from build123d import *

# Parameters (mm, degrees)
F1_DEPTH = 14.224
F2_DEPTH = 7.874
F3_DEPTH = 12.7


with BuildPart() as f1:
    # F0 (on Front) → F1 (new body, symmetric)
    with BuildSketch(Plane.XZ):
        Polygon((22.958146, 14.2875), (-45.974, 14.2875), (-52.324, 14.2875), (-52.324, -14.2875), (-45.974, -14.2875), (22.958146, -14.2875), align=None)
    extrude(amount=F1_DEPTH, both=True)

    # F0 (on Front) → F2 (join, symmetric)
    with BuildSketch(Plane.XZ):
        Polygon((17.272, 25.2095), (17.272, 42.7355), (-45.974, 42.7355), (-45.974, 14.2875), (22.958146, 14.2875), (32.52297, 14.2875), (40.125151, 25.2095), align=None)
        with BuildLine():
            Line((0, 22.1615), (-21.336, 22.1615))
            ThreePointArc((-21.336, 22.1615), (-27.686, 28.5115), (-21.336, 34.8615))
            Line((-21.336, 34.8615), (0, 34.8615))
            ThreePointArc((0, 34.8615), (6.35, 28.5115), (0, 22.1615))
        make_face(mode=Mode.SUBTRACT)
        Polygon((32.52297, -14.2875), (22.958146, -14.2875), (-45.974, -14.2875), (-45.974, -42.7355), (17.272, -42.7355), (17.272, -25.365404), (40.233667, -25.365404), align=None)
        with BuildLine():
            Line((0, -34.8615), (-21.336, -34.8615))
            ThreePointArc((-21.336, -34.8615), (-27.686, -28.5115), (-21.336, -22.1615))
            Line((-21.336, -22.1615), (0, -22.1615))
            ThreePointArc((0, -22.1615), (6.35, -28.5115), (0, -34.8615))
        make_face(mode=Mode.SUBTRACT)
    extrude(amount=F2_DEPTH, both=True)

    # F0 (on Front) → F3 (join, symmetric)
    with BuildSketch(Plane.XZ):
        Polygon((40.125151, 25.2095), (52.324, 42.7355), (17.272, 42.7355), (17.272, 25.2095), align=None)
        Polygon((52.324, -42.7355), (40.233667, -25.365404), (17.272, -25.365404), (17.272, -42.7355), align=None)
    extrude(amount=F3_DEPTH, both=True)


solid = f1.part
Design review of the part built by this model. Coordinates are the model's own, in mm. A direction names the side the tool comes from. Give positions to 0.01 mm unless a question says otherwise; leave off trailing zeros. Loops run counter-clockwise (first coordinate to the right, second up) from the corner with the lowest first, then second, coordinate; pieces in that order, holes last. Notation, with made-up numbers: M -39,71 L 12,71 A6 cw 12,76 Z; hole C 76,62.25 d10. An arc over 180 degrees is marked long. Write item = value, one per line.
Q1. We need section A-A (x = 30.5). Give the boundary of the cut face in (y, z), plus the area to 3 significant figures.
Output values:
outline = M -12.7,-42.74 L 12.7,-42.74 L 12.7,-25.37 L 7.87,-25.37 L 7.87,-14.29 L -7.87,-14.29 L -7.87,-25.37 L -12.7,-25.37 Z; M -12.7,25.21 L -7.87,25.21 L -7.87,14.29 L 7.87,14.29 L 7.87,25.21 L 12.7,25.21 L 12.7,42.74 L -12.7,42.74 Z
area = 1,230 mm^2
Q2. To check wall thickness, follow line 1 (Z direction, x = -20, y = 5.5); line 2 (Z direction, x = 35, y = -10); line 3 (Z direction, x = 37, y = -6.25). State the ranges of each line that lie inside material, in increasing order. Write a range as [from, to].
Output values:
line_1 = [-42.74, -34.86], [-22.16, 22.16], [34.86, 42.74]
line_2 = [-42.74, -25.37], [25.21, 42.74]
line_3 = [-42.74, -20.72], [20.72, 42.74]
Q3. Insertion check: pin 1 (9 mm diameter, centred on x = 33.5, z = 34.5, fed in from -Y); pin 2 (3 mm diameter, centred on x = -22, z = 14.5, fed in from +Y); pin 3 (14 mm diameter, centred on x = 27, z = -32, fed in from +Y); pin 4 (6 mm diameter, centred on y = -2, z = 16.5, fed in from +X). Each pin has a flat end and moves straight along its axis. Give the tip position at first contact, or say it passes through.
Output values:
pin_1 = -12.7
pin_2 = 14.22
pin_3 = 12.7
pin_4 = 36.15
Q4. We need section C-C (y = 4.5). Give the boundary of the cut face in (x, z), plus the area to 3 significant figures.
Output values:
outline = M -52.32,-14.29 L -45.97,-14.29 L -45.97,-42.74 L 52.32,-42.74 L 32.52,-14.29 L 22.96,-14.29 L 22.96,14.29 L 32.52,14.29 L 52.32,42.74 L -45.97,42.74 L -45.97,14.29 L -52.32,14.29 Z; hole M -21.34,-34.86 L 0,-34.86 A6.35 ccw 0,-22.16 L -21.34,-22.16 A6.35 ccw Z; hole M -21.34,22.16 L 0,22.16 A6.35 ccw 0,34.86 L -21.34,34.86 A6.35 ccw Z
area = 6,390 mm^2
Q5. For faces 4 (the flat face through (29, -10, 25.21)), 5 (the flat face through (-11, 0, 22.162)), 6 (the flat face through (28, 0, 14.288)), list the 3-axis set-ups (+Z, -Z, +X, -X, +Y, -Y) from which the entire face can be reached by the end or side of a thin tool; tool diameter is ignored.
Output values:
face_4 = +X, -X, -Y
face_5 = +Y, -Y
face_6 = +X, +Y, -Y
Q6. Draft analysis for pull direction X (two halves, no side actions). For faces 1 (the flat face through (22.958, 0, 0)), 2 (the cylindrical face through (-27.684, 0.11, 28.372)), 3 (the flat face through (-14, -10, 14.288)), state which applies: +X half, -X half, draft (parallel to the pull), parting line (faces both ways), or undercut.
Output values:
face_1 = +X half
face_2 = undercut
face_3 = draft
Q7. We need section D-D (x = -34). Give the boundary of the cut face in (y, z).
Output values:
outline = M -14.22,-14.29 L -7.87,-14.29 L -7.87,-42.74 L 7.87,-42.74 L 7.87,-14.29 L 14.22,-14.29 L 14.22,14.29 L 7.87,14.29 L 7.87,42.74 L -7.87,42.74 L -7.87,14.29 L -14.22,14.29 Z
Q8. We need section B-B (y = -10.5). Give the boundary of the cut face in (x, z).
Output values:
outline = M -52.32,-14.29 L 22.96,-14.29 L 22.96,14.29 L -52.32,14.29 Z; M 17.27,-42.74 L 52.32,-42.74 L 40.23,-25.37 L 17.27,-25.37 Z; M 17.27,25.21 L 40.13,25.21 L 52.32,42.74 L 17.27,42.74 Z
